```python
from build123d import *

# Parameters (mm, degrees)
IZIM1_R                     = 1.5
IZIM1_R_2                   = 22.5
Y_KSEKLIK_EKSTR_ZYON1_DEPTH = 10


with BuildPart() as part:
    # Çizim1 → Yükseklik-Ekstrüzyon1 (new body)
    with BuildSketch(Plane.XY.offset(10)):
        with BuildLine():
            Line((3, -38), (47, -38))
            ThreePointArc((47, -38), (49.121320344, -37.121320344), (50, -35))
            Line((50, -35), (50, 55))
            ThreePointArc((50, 55), (49.121320344, 57.121320344), (47, 58))
            Line((47, 58), (39.5, 58))
            Line((39.5, 58), (39.5, 69))
            Line((39.5, 69), (10, 69))
            Line((10, 69), (10, 58))
            Line((10, 58), (3, 58))
            ThreePointArc((3, 58), (0.878679656, 57.121320344), (0, 55))
            Line((0, 55), (0, -35))
            ThreePointArc((0, -35), (0.878679656, -37.121320344), (3, -38))
        make_face()
        with Locations(Location((15, 64, 0), (0, 0, 180))):
            Circle(IZIM1_R, mode=Mode.SUBTRACT)
        with Locations((25, -8)):
            Circle(IZIM1_R_2, mode=Mode.SUBTRACT)
        with Locations(Location((35, 64, 0), (0, 0, 180))):
            Circle(IZIM1_R, mode=Mode.SUBTRACT)
    extrude(amount=-Y_KSEKLIK_EKSTR_ZYON1_DEPTH)


solid = part.part
```
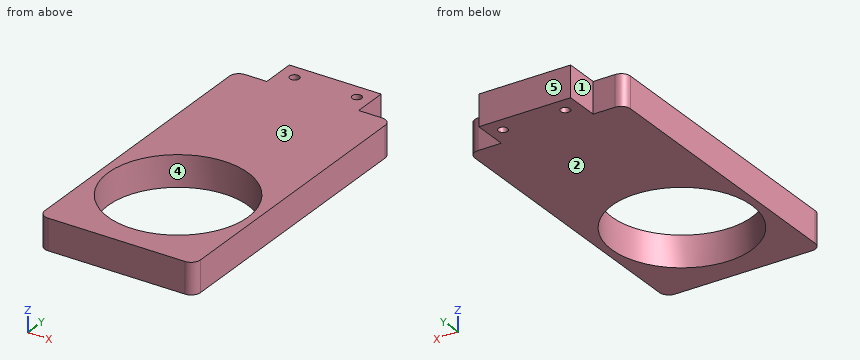
Can you work these out from the model? Positions are in its coordinate system, mm. Face numbers are marked on the shaded views. A direction names the side the tool comes from. Coordinates: 2 decimals unless noted, no trailing zeros. Loops run counter-clockwise (first coordinate to the right, second up) from the corner with the lowest first, then second, coordinate; pieces in that order, holes last.
Item 1: I'm going to push a flat-ended pin straight in: pin 1 (4 mm diameter, centred on x = 42.5, z = 4.5, fed in from +Y). Where does the tip first touch, or does it pass through?
Answers below:
pin 1: stops at y = 58
Item 2: Which directions (+Z, -Z, +X, -X, +Y, -Y) give clear straight access to the entire face, cutting with the end or side of a thin tool? Please do the marked faces 1 and 2.
Answers below:
face 1: +Z, -Z, -X, +Y
face 2: -Z, +X, -X, +Y, -Y
Item 3: Please list where these lines run through material, in increasing order: L1, parallel to X at y = 64, z = 7.25; L2, parallel to Y at x = 35, z = 6.25; L3, parallel to Y at x = 14.5, z = 7.5.
Answers below:
L1: x = 10 to 13.5, 16.5 to 33.5, 36.5 to 39.5
L2: y = -38 to -28.16, 12.16 to 62.5, 65.5 to 69
L3: y = -38 to -27.9, 11.9 to 62.59, 65.41 to 69
Item 4: Suppose I cut it at C-C (x = 25). Please give me the cut outline in (y, z), then the cut area to 3 significant figures.
Answers below:
outline: (-38, 0) - (-30.5, 0) - (-30.5, 10) - (-38, 10) - close; (14.5, 0) - (69, 0) - (69, 10) - (14.5, 10) - close
area: 620 mm2
Item 5: Suppose I cut it at A-A (y = -8). Please give me the cut outline in (x, z), then the cut area to 3 significant figures.
Answers below:
outline: (0, 0) - (2.5, 0) - (2.5, 10) - (0, 10) - close; (47.5, 0) - (50, 0) - (50, 10) - (47.5, 10) - close
area: 50.0 mm2
Item 6: Suppose I cut it at D-D (z = 1.25). Please give me the cut outline in (x, y), then the cut area to 3 significant figures.
Answers below:
outline: (0, -35) arc R3 ccw to (3, -38) - (47, -38) arc R3 ccw to (50, -35) - (50, 55) arc R3 ccw to (47, 58) - (39.5, 58) - (39.5, 69) - (10, 69) - (10, 58) - (3, 58) arc R3 ccw to (0, 55) - close; hole circle Ø45 at (25, -8); hole circle Ø3 at (15, 64); hole circle Ø3 at (35, 64)
area: 3,510 mm2
Item 7: Suppose I cut it at B-B (y = 64). Please give me the cut outline in (x, z), then the cut area to 3 significant figures.
Answers below:
outline: (10, 0) - (13.5, 0) - (13.5, 10) - (10, 10) - close; (16.5, 0) - (33.5, 0) - (33.5, 10) - (16.5, 10) - close; (36.5, 0) - (39.5, 0) - (39.5, 10) - (36.5, 10) - close
area: 235 mm2
Item 8: If we mould it in two halves opening along Y, with no side actions, what happens to the marked faces 3, 4 and 5? For each: released by +Y, released by -Y, zero draft, split by the parting line, or undercut.
Answers below:
face 3: zero draft
face 4: undercut
face 5: released by +Y
